Build history of the part. All positions in model axes, mm. A direction names the side the tool comes from. Coordinates: 2 decimals unless noted, no trailing zeros. Loops run counter-clockwise (first coordinate to the right, second up) from the corner with the lowest first, then second, coordinate; pieces in that order, holes last.
(1) Tool access for faces 5 (the face through (-75.53, 57.57, 6.44)), 6 (the face through (82.593, -2.864, 6.261)): list every direction of +Z, -Z, +X, -X, +Y, -Y with a clear straight run to the whole face (end or side of a thin tool).
(2) Slice it at C-C (y = 21.5). Give the cut face in (x, z), and give its area (3 significant figures).
(3) Flat gauge pins, fed straight in: P1, Ø1, axis at x = 26.5, z = 11, coming from the -Y side; P2, Ø3, axis at y = 81.5, z = 9, coming from the -X side; P3, Ø1, axis at y = 58, z = 8, coming from the -X side. Where does each tip first touch, or does it go through?
(4) Two-plate mould, pull along Y, no slides. Class faces 1 (the face through (34.325, -33.93, 6.439)), 2 (the face through (-2, 2, 0)), 3 (the face through (-103.728, 73.277, 6.261)), 4 (the face through (-1.013, -82.555, 6.261)): pulls with the +Y half, pulls with the -Y half, needs draft (parallel to the pull), parting line crosses it, or undercut.
(5) Slice it at B-B (y = -71.5). Give the cut face in (x, z), and give its area (3 significant figures).
(6) Wall check: L1, parallel to X at y = -35, z = 3; L2, parallel to Y at x = -72, z = 6.5; L3, parallel to X at y = 54.5, z = 12. Give the ranges that are in metal, low to high.
(7) Slice it at A-A (x = -48). Give the cut face in (y, z), and give its area (3 significant figures).
(8) Slice it at D-D (x = -6). Give the cut face in (y, z).
from build123d import *

# Parameters (mm, degrees)
F1_DEPTH = 12.7
F3_R     = 5.08
F4_DEPTH = 25.4


with BuildPart() as f1:
    # F0 (on Top) → F1 (new body)
    with BuildSketch(Plane.XY):
        with BuildLine():
            ThreePointArc((108.74375, -65.6033294577), (82.55, 0), (108.74375, 65.6033294577))
            ThreePointArc((108.74375, 65.6033294577), (89.8025612107, 89.8025612107), (65.6033294577, 108.74375))
            ThreePointArc((65.6033294577, 108.74375), (0, 82.55), (-65.6033294577, 108.74375))
            ThreePointArc((-65.6033294577, 108.74375), (-89.8025612107, 89.8025612107), (-108.74375, 65.6033294577))
            ThreePointArc((-108.74375, 65.6033294577), (-82.55, 0), (-108.74375, -65.6033294577))
            ThreePointArc((-108.74375, -65.6033294577), (-89.8025612107, -89.8025612107), (-65.6033294577, -108.74375))
            ThreePointArc((-65.6033294577, -108.74375), (0, -82.55), (65.6033294577, -108.74375))
            ThreePointArc((65.6033294577, -108.74375), (89.8025612107, -89.8025612107), (108.74375, -65.6033294577))
        make_face()
    extrude(amount=F1_DEPTH)

    # F3
    f3_edges = [f1.edges().sort_by_distance(p)[0] for p in [
        (65.603329, 108.74375, 6.35),
        (108.74375, 65.603329, 6.35),
    ]]
    fillet(f3_edges, radius=F3_R)

    # F2 (on face) → F4 (cut)
    with BuildSketch(Plane.XY.offset(12.7)):
        with BuildLine():
            Line((105.9670222286, 88.0065099865), (96.9867661075, 96.9867661075))
            Line((96.9867661075, 96.9867661075), (88.0065099865, 105.9670222286))
            Line((88.0065099865, 105.9670222286), (34.1249732601, 52.0854855022))
            ThreePointArc((34.1249732601, 52.0854855022), (34.1249732601, 34.1249732601), (52.0854855022, 34.1249732601))
            Line((52.0854855022, 34.1249732601), (105.9670222286, 88.0065099865))
        make_face()
        with BuildLine():
            ThreePointArc((-52.0854855022, 34.1249732601), (-34.1249732601, 34.1249732601), (-34.1249732601, 52.0854855022))
            Line((-34.1249732601, 52.0854855022), (-88.0065099865, 105.9670222286))
            Line((-88.0065099865, 105.9670222286), (-96.9867661075, 96.9867661075))
            Line((-96.9867661075, 96.9867661075), (-105.9670222286, 88.0065099865))
            Line((-105.9670222286, 88.0065099865), (-52.0854855022, 34.1249732601))
        make_face()
        with BuildLine():
            Line((-88.0065099865, -105.9670222286), (-34.1249732601, -52.0854855022))
            ThreePointArc((-34.1249732601, -52.0854855022), (-34.1249732601, -34.1249732601), (-52.0854855022, -34.1249732601))
            Line((-52.0854855022, -34.1249732601), (-105.9670222286, -88.0065099865))
            Line((-105.9670222286, -88.0065099865), (-96.9867661075, -96.9867661075))
            Line((-96.9867661075, -96.9867661075), (-88.0065099865, -105.9670222286))
        make_face()
        with BuildLine():
            Line((34.1249732601, -52.0854855022), (88.0065099865, -105.9670222286))
            Line((88.0065099865, -105.9670222286), (96.9867661075, -96.9867661075))
            Line((96.9867661075, -96.9867661075), (105.9670222286, -88.0065099865))
            Line((105.9670222286, -88.0065099865), (52.0854855022, -34.1249732601))
            ThreePointArc((52.0854855022, -34.1249732601), (34.1249732601, -34.1249732601), (34.1249732601, -52.0854855022))
        make_face()
    extrude(amount=-F4_DEPTH, mode=Mode.SUBTRACT)


solid = f1.part
Response values:
1. face 5: +Z, -Z
1. face 6: +Z, -Z, +X
2. outline: (-85.01, 0) - (85.01, 0) - (85.01, 12.7) - (-85.01, 12.7) - close
2. area: 2,160 mm2
3. P1: stops at y = -86.46
3. P2: stops at x = -98.64
3. P3: stops at x = -102.63
4. face 1: undercut
4. face 2: needs draft
4. face 3: pulls with the +Y half
4. face 4: pulls with the -Y half
5. outline: (-104.96, 0) - (-89.46, 0) - (-89.46, 12.7) - (-104.96, 12.7) - close; (-53.54, 0) - (53.54, 0) - (53.54, 12.7) - (-53.54, 12.7) - close; (89.46, 0) - (104.96, 0) - (104.96, 12.7) - (89.46, 12.7) - close
5. area: 1,750 mm2
6. L1: x = -89.21 to -52.96, -33.33 to 33.33, 52.96 to 89.21
6. L2: y = -104.62 to -89.96, -54.04 to 54.04, 89.96 to 104.62
6. L3: x = -99.68 to -72.46, -36.54 to 36.54, 72.46 to 99.68
7. outline: (-95.53, 0) - (-65.96, 0) - (-65.96, 12.7) - (-95.53, 12.7) - close; (-31.39, 0) - (31.39, 0) - (31.39, 12.7) - (-31.39, 12.7) - close; (65.96, 0) - (95.53, 0) - (95.53, 12.7) - (65.96, 12.7) - close
7. area: 1,550 mm2
8. outline: (-82.74, 0) - (82.74, 0) - (82.74, 12.7) - (-82.74, 12.7) - close
